from build123d import *

# Parameters (mm, degrees)
SKETCH1_R               = 4.7625
BOSS_EXTRUDE1_DEPTH     = 66.675
SKETCH1_4_R             = 9.999999939
SKETCH1_4_R_2           = 3.175
BOSS_EXTRUDE2_DEPTH     = 4.7625
FILLET1_R               = 3.175
SKETCH3_R               = 0.899999978
CUT_EXTRUDE2_DEPTH      = 10.999999939
CUT_EXTRUDE2_DEPTH_BACK = 10.999999939
SKETCH4_R               = 0.899999978
CUT_EXTRUDE3_DEPTH      = 14.927284721
CUT_EXTRUDE3_DEPTH_BACK = 14.927284721
SKETCH5_R               = 0.899999978
CUT_EXTRUDE4_DEPTH      = 14.927284721
CUT_EXTRUDE4_DEPTH_BACK = 14.927284721
CUT_EXTRUDE5_DEPTH      = 72.4375001
BOSS_EXTRUDE3_DEPTH     = 4.7625
CIRPATTERN1_COUNT       = 4


with BuildPart() as part:
    # Sketch1 → Boss-Extrude1 (new body)
    with BuildSketch(Plane.XY):
        Circle(SKETCH1_R)
    extrude(amount=BOSS_EXTRUDE1_DEPTH)

    # Sketch1<4> → Boss-Extrude2 (add)
    with BuildSketch(Plane.XY):
        Circle(SKETCH1_4_R)
        Circle(SKETCH1_4_R_2, mode=Mode.SUBTRACT)
    extrude(amount=-BOSS_EXTRUDE2_DEPTH)

    # Fillet1
    fillet1_edges = [part.edges().sort_by_distance(p)[0] for p in [
        (-3.175, 0, 0),
    ]]
    fillet(fillet1_edges, radius=FILLET1_R)

    # Sketch3 → Cut-Extrude2 (cut, two sides)
    with BuildSketch(Plane(origin=(0, 0, 0), x_dir=(0, 0, -1), z_dir=(1, 0, 0))) as cut_extrude2_sk:
        with Locations((-38.89375, 0)):
            Circle(SKETCH3_R)
    extrude(amount=CUT_EXTRUDE2_DEPTH, mode=Mode.SUBTRACT)
    extrude(cut_extrude2_sk.sketch, amount=-CUT_EXTRUDE2_DEPTH_BACK, mode=Mode.SUBTRACT)

    # Sketch4 → Cut-Extrude3 (cut, two sides)
    with BuildSketch(Plane(origin=(0, 0, 0), x_dir=(0, 0, -1), z_dir=(0.573576436, 0.819152044, 0))) as cut_extrude3_sk:
        with Locations((-53.18125, 0)):
            Circle(SKETCH4_R)
    extrude(amount=CUT_EXTRUDE3_DEPTH, mode=Mode.SUBTRACT)
    extrude(cut_extrude3_sk.sketch, amount=-CUT_EXTRUDE3_DEPTH_BACK, mode=Mode.SUBTRACT)

    # Sketch5 → Cut-Extrude4 (cut, two sides)
    with BuildSketch(Plane(origin=(0, 0, 0), x_dir=(0, 0, -1), z_dir=(-0.573576436, 0.819152044, 0))) as cut_extrude4_sk:
        with Locations((-24.60625, 0)):
            Circle(SKETCH5_R)
    extrude(amount=CUT_EXTRUDE4_DEPTH, mode=Mode.SUBTRACT)
    extrude(cut_extrude4_sk.sketch, amount=-CUT_EXTRUDE4_DEPTH_BACK, mode=Mode.SUBTRACT)

    # Sketch6 → Cut-Extrude5 (cut, through all)
    with BuildSketch(Plane(origin=(0, 0, -4.7625), x_dir=(-1, 0, 0), z_dir=(0, 0, -1))):
        with BuildLine():
            ThreePointArc((0, 6.249999819), (1.050000059, 7.299999878), (0, 8.349999937))
            ThreePointArc((0, 8.349999937), (-2.275161332, 8.034061231), (-4.378152237, 7.11015344))
            ThreePointArc((-4.378152237, 7.11015344), (-6.820637013, 3.874042781), (-3.080152041, 5.438304988))
            ThreePointArc((-3.080152041, 5.438304988), (-1.592653846, 6.043670364), (0, 6.249999819))
        make_face()
    cut_extrude5 = extrude(amount=-CUT_EXTRUDE5_DEPTH, mode=Mode.SUBTRACT)

    # Sketch7 → Boss-Extrude3 (add)
    with BuildSketch(Plane(origin=(0, 0, -4.7625), x_dir=(-1, 0, 0), z_dir=(0, 0, -1))):
        with BuildLine():
            ThreePointArc((-0.506000912, 6.379965531), (-0.809595225, 6.348586667), (-1.111348298, 6.302769396))
            Line((-1.111348298, 6.302769396), (-1.329589914, 6.106937727))
            ThreePointArc((-1.329589914, 6.106937727), (-0.963002055, 6.175364344), (-0.592985752, 6.221805657))
            Line((-0.592985752, 6.221805657), (-0.506000912, 6.379965531))
        make_face()
        with BuildLine():
            Line((-1.632295539, 8.188901649), (-1.423915054, 8.075423558))
            ThreePointArc((-1.423915054, 8.075423558), (-0.999751281, 8.138826519), (-0.57285269, 8.179965741))
            Line((-0.57285269, 8.179965741), (-0.666214637, 8.323380143))
            ThreePointArc((-0.666214637, 8.323380143), (-1.151220385, 8.270259402), (-1.632295539, 8.188901649))
        make_face()
    boss_extrude3 = extrude(amount=-BOSS_EXTRUDE3_DEPTH)

    # CirPattern1: Cut-Extrude5, Boss-Extrude3 ×4 about axis
    cirpattern1_axis = Axis((0, 0, 0), (0, 0, 1))
    for i in range(1, CIRPATTERN1_COUNT):
        add(cut_extrude5.rotate(cirpattern1_axis, i * 360 / CIRPATTERN1_COUNT), mode=Mode.SUBTRACT)
        add(boss_extrude3.rotate(cirpattern1_axis, i * 360 / CIRPATTERN1_COUNT))


solid = part.part
Input: part model. Units: mm. Frame: model coordinates. A direction names the side the tool comes from. Coordinates: 2 decimals unless noted, no trailing zeros. Order: outer loops, then holes, each group sorted by start corner. A loop starts at its lowest first (then second) coordinate and runs counter-clockwise, first axis right, second up. Notation, with made-up numbers: M 2.5,4 L 31.5,4 A16 ccw 31.5,26 Z; hole C -35.5,74 d10. An arc over 180 degrees is marked long. One line per question, with ' | ' between items.
Item 1: Section A-A (z = 56.5). Output: boundary loops of the cut face in (x, y) (1 decimal), then the cut area to 3 significant figures.
Geometry results:
outline: C 0,0 d9.5 | area: 71.3 mm^2
Item 2: Ray query, line 1 along Z through (x, y) = (3.6, 0) (1 decimal); line 2 along X through (y, z) = (-7.5, -1.5); line 3 along Z through (x, y) = (-4.5, -0.5) (1 decimal). Return the intervals inside material, ascending.
Geometry results:
line 1: z = -4.8 to 38, 39.8 to 66.7 | line 2: x = -6.61 to -3.67, 1.03 to 6.61 | line 3: z = -4.8 to 38.1, 39.6 to 66.7
Item 3: Reachability of faces 5 (the cylindrical face through (-0.69, -3.1, -3.96)), 6 (the cylindrical face through (7.28, 1.05, -2.41)), 7 (the flat face through (0, 0, 66.675)), 8 (the cylindrical face through (-3.78, -2.9, 32.87)) from +Z, -Z, +X, -X, +Y, -Y: full face, straight path, thin tool, end or side. Return the list, or none.
Geometry results:
face 5: -Z | face 6: +Z, -Z | face 7: +Z, +X, -X, +Y, -Y | face 8: +Z
Item 4: Draft query along X for faces 1 (the flat face through (-2.4, 2.4, -4.762)), 2 (the cylindrical face through (-7.28, -1.05, -2.41)), 3 (the cylindrical face through (4.614, -8.872, -2.348)), 4 (the cylindrical face through (-7.78, 3.03, -2.41)). Return one class per face: released by +X, released by -X, zero draft, split by the parting line, or undercut.
Geometry results:
face 1: zero draft | face 2: undercut | face 3: split by the parting line | face 4: undercut
Item 5: Pin query (flat end, axial travel): pin 1 (2 mm diameter, centred on x = -5, y = -7.5, fed in from +Z); pin 2 (2.5 mm diameter, centred on y = 0, z = 38.89, fed in from -X); pin 3 (2 mm diameter, centred on x = -3, z = 11, fed in from +Y); pin 4 (1.1 mm diameter, centred on y = 0, z = 38.89, fed in from -X). Return the tip coordinate at first contact, or that it passes through.
Geometry results:
pin 1: stops at z = 0 | pin 2: stops at x = -4.76 | pin 3: stops at y = 4.32 | pin 4: passes through
